Geometry: final body of the model. Coordinates: model frame, mm. A direction names the side the tool comes from. Round coordinates to 2 decimals unless told otherwise and drop trailing zeros. Order: outer loops, then holes, each group sorted by start corner. A loop starts at its lowest first (then second) coordinate and runs counter-clockwise, first axis right, second up. Notation, with made-up numbers: (-40, 84.5) -> (-14, 84.5) arc R17 cw to (-14, 93.5) -> close; hole circle Ø3 at (75.25, 48). An arc over 180 degrees is marked (long way). Put each result on its own line as item: value.
```python
from build123d import *

# Parameters (mm, degrees)
SKETCH1_R           = 50.8
SKETCH1_R_2         = 44.45
BOSS_EXTRUDE1_DEPTH = 38.1
SKETCH1_4_R         = 44.45
SKETCH1_4_R_2       = 6.35
SKETCH1_4_R_3       = 19.05
BOSS_EXTRUDE3_DEPTH = 25.4
SKETCH1_5_R         = 19.05
SKETCH1_5_R_2       = 12.7
BOSS_EXTRUDE4_DEPTH = 57.15
SKETCH1_6_R         = 12.7
SKETCH1_6_R_2       = 7.112
BOSS_EXTRUDE5_DEPTH = 76.2


with BuildPart() as part:
    # Sketch1 → Boss-Extrude1 (new body)
    with BuildSketch(Plane(origin=(0, 0, 0), x_dir=(1, 0, 0), z_dir=(0, 1, 0))):
        Circle(SKETCH1_R)
        Circle(SKETCH1_R_2, mode=Mode.SUBTRACT)
    extrude(amount=BOSS_EXTRUDE1_DEPTH)

    # Sketch1<4> → Boss-Extrude3 (add)
    with BuildSketch(Plane(origin=(0, 0, 0), x_dir=(1, 0, 0), z_dir=(0, 1, 0))):
        Circle(SKETCH1_4_R)
        with Locations((29.337, 0)):
            Circle(SKETCH1_4_R_2, mode=Mode.SUBTRACT)
        with Locations((0, -29.337)):
            Circle(SKETCH1_4_R_2, mode=Mode.SUBTRACT)
        with Locations((-29.337, 0)):
            Circle(SKETCH1_4_R_2, mode=Mode.SUBTRACT)
        with Locations((0, 29.337)):
            Circle(SKETCH1_4_R_2, mode=Mode.SUBTRACT)
        Circle(SKETCH1_4_R_3, mode=Mode.SUBTRACT)
    extrude(amount=BOSS_EXTRUDE3_DEPTH)

    # Sketch1<5> → Boss-Extrude4 (add)
    with BuildSketch(Plane(origin=(0, 0, 0), x_dir=(1, 0, 0), z_dir=(0, 1, 0))):
        Circle(SKETCH1_5_R)
        Circle(SKETCH1_5_R_2, mode=Mode.SUBTRACT)
    extrude(amount=BOSS_EXTRUDE4_DEPTH)

    # Sketch1<6> → Boss-Extrude5 (add)
    with BuildSketch(Plane(origin=(0, 0, 0), x_dir=(1, 0, 0), z_dir=(0, 1, 0))):
        Circle(SKETCH1_6_R)
        Circle(SKETCH1_6_R_2, mode=Mode.SUBTRACT)
    extrude(amount=BOSS_EXTRUDE5_DEPTH)


solid = part.part
```
1. Material intervals for probe 1 along Z at (x, y) = (0, 32.25); probe 2 along Z at (x, y) = (0, 12); probe 3 along Z at (x, y) = (8, 26), sorted ascending.
Ans:
probe 1: -50.8 to -44.45, -19.05 to -7.11, 7.11 to 19.05, 44.45 to 50.8
probe 2: -50.8 to -35.69, -22.99 to -7.11, 7.11 to 22.99, 35.69 to 50.8
probe 3: -50.17 to -43.72, -17.29 to 17.29, 43.72 to 50.17
2. Cut plane C-C on y = 36. Return loops of the section in (x, z), and give its area (3 significant figures).
Ans:
outline: circle Ø101.6 at (0, 0); circle Ø38.1 at (0, 0); hole circle Ø88.9 at (0, 0); hole circle Ø14.22 at (0, 0)
area: 2,880 mm²
3. Contact query for flat-ended pins moving along their axis: P1, Ø7.5, axis at x = 29.337, z = 0, coming from the -Y side; P2, Ø2, axis at x = 9.5, y = 31.5, coming from the +Z side; P3, Ø2, axis at x = -5, z = -11, coming from the -Y side; P4, Ø1, axis at x = -23.5, z = -34, coming from the +Y side. Output: stop coordinate, or through.
Ans:
P1: through
P2: z = 50.08
P3: y = 0
P4: y = 25.4
4. Cut plane B-B on x = 0. Return loops of the section in (y, z), and give its area (3 significant figures).
Ans:
outline: (0, -50.8) -> (38.1, -50.8) -> (38.1, -44.45) -> (25.4, -44.45) -> (25.4, -35.69) -> (0, -35.69) -> close; (0, -22.99) -> (25.4, -22.99) -> (25.4, -19.05) -> (57.15, -19.05) -> (57.15, -12.7) -> (76.2, -12.7) -> (76.2, -7.11) -> (0, -7.11) -> close; (0, 7.11) -> (76.2, 7.11) -> (76.2, 12.7) -> (57.15, 12.7) -> (57.15, 19.05) -> (25.4, 19.05) -> (25.4, 22.99) -> (0, 22.99) -> close; (0, 35.69) -> (25.4, 35.69) -> (25.4, 44.45) -> (38.1, 44.45) -> (38.1, 50.8) -> (0, 50.8) -> close
area: 2,710 mm²
5. Cut plane A-A on z = 0. Return loops of the section in (x, y), and give its area (3 significant figures).
Ans:
outline: (-50.8, 0) -> (-35.69, 0) -> (-35.69, 25.4) -> (-44.45, 25.4) -> (-44.45, 38.1) -> (-50.8, 38.1) -> close; (-22.99, 0) -> (-7.11, 0) -> (-7.11, 76.2) -> (-12.7, 76.2) -> (-12.7, 57.15) -> (-19.05, 57.15) -> (-19.05, 25.4) -> (-22.99, 25.4) -> close; (7.11, 0) -> (22.99, 0) -> (22.99, 25.4) -> (19.05, 25.4) -> (19.05, 57.15) -> (12.7, 57.15) -> (12.7, 76.2) -> (7.11, 76.2) -> close; (35.69, 0) -> (50.8, 0) -> (50.8, 38.1) -> (44.45, 38.1) -> (44.45, 25.4) -> (35.69, 25.4) -> close
area: 2,710 mm²
6. Draft query along Z for faces 3 (the face through (-11.012, 18.783, 49.592)), 4 (the face through (-1.542, 37.567, 6.943)), 5 (the face through (11, 0, -1)). Return one class per face: +Z half, -Z half, draft (parallel to the pull), parting line (faces both ways), or undercut.
Ans:
face 3: parting line
face 4: undercut
face 5: draft
7. Cut plane D-D on z = 25. Return loops of the section in (x, y), and give its area (3 significant figures).
Ans:
outline: (-44.22, 0) -> (-4.64, 0) -> (-4.64, 25.4) -> (-36.75, 25.4) -> (-36.75, 38.1) -> (-44.22, 38.1) -> close; (4.64, 0) -> (44.22, 0) -> (44.22, 38.1) -> (36.75, 38.1) -> (36.75, 25.4) -> (4.64, 25.4) -> close
area: 2,200 mm²
8. Set-up query: faces 1 (the face through (4, 57.15, 12.4)), 2 (the face through (35.203, 12.522, 2.432)). Return all of +Z, -Z, +X, -X, +Y, -Y with unobstructed straight access to the full face (end or side cutting, diameter ignored); none if empty.
Ans:
face 1: +Y
face 2: +Y, -Y
